Design review of the part built by this model. Coordinates are the model's own, in mm. A direction names the side the tool comes from. Coordinates: 2 decimals unless noted, no trailing zeros. Loops run counter-clockwise (first coordinate to the right, second up) from the corner with the lowest first, then second, coordinate; pieces in that order, holes last. Notation, with made-up numbers: (-4, 4.25) - (5, 4.25) arc R8 cw to (5, 11.25) - close; hole circle Ø8 at (44, 43.25). An arc over 180 degrees is marked (long way). One line per question, with ' | ' between items.
from build123d import *

# Parameters (mm, degrees)
F1_DEPTH = 76.2
F2_R     = 12.7
F3_DEPTH = 76.201
F5_DEPTH = 25.401
F6_R     = 38.1
F7_R     = 19.05
F8_DEPTH = 6.35


with BuildPart() as f1:
    # F0 (on Front) → F1 (new body, symmetric)
    with BuildSketch(Plane.XZ):
        Polygon((-76.2, 0), (0, 0), (0, 152.4), (-25.4, 152.4), (-25.4, 25.4), (-76.2, 25.4), align=None)
    extrude(amount=F1_DEPTH, both=True)

    # F2 (on face) → F3 (cut, through all)
    with BuildSketch(Plane.YZ):
        with Locations((0, 101.6)):
            Circle(F2_R)
    extrude(amount=-F3_DEPTH, mode=Mode.SUBTRACT)

    # F4 (on face) → F5 (cut, through all)
    with BuildSketch(Plane.XY.offset(25.4)):
        with BuildLine():
            ThreePointArc((-63.5, -6.35), (-59.009872, -4.490128), (-57.15, 0))
            ThreePointArc((-57.15, 0), (-59.009872, 4.490128), (-63.5, 6.35))
            ThreePointArc((-63.5, 6.35), (-69.85, 0), (-63.5, -6.35))
        make_face()
        with BuildLine():
            ThreePointArc((-63.5, -6.35), (-69.85, 0), (-63.5, 6.35))
            Line((-63.5, 6.35), (-76.2, 6.35))
            Line((-76.2, 6.35), (-76.2, -6.35))
            Line((-76.2, -6.35), (-63.5, -6.35))
        make_face()
    extrude(amount=-F5_DEPTH, mode=Mode.SUBTRACT)

    # F6
    f6_edges = [f1.edges().sort_by_distance(p)[0] for p in [
        (-12.7, -76.2, 152.4),
        (-12.7, 76.2, 152.4),
    ]]
    fillet(f6_edges, radius=F6_R)

    # F7 (on face) → F8 (cut)
    with BuildSketch(Plane(origin=(-25.4, 0, 0), x_dir=(0, -1, 0), z_dir=(-1, 0, 0))):
        with Locations((0, 101.6)):
            Circle(F7_R)
    extrude(amount=-F8_DEPTH, mode=Mode.SUBTRACT)


solid = f1.part
Q1. Take a section at B-B (y = 23). Give the boundary of the cut face in (x, z), plus the area to 3 significant figures.
Returned:
outline: (-76.2, 0) - (0, 0) - (0, 152.4) - (-25.4, 152.4) - (-25.4, 25.4) - (-76.2, 25.4) - close | area: 5,160 mm²
Q2. For pin 1 (1.5 mm diameter, centred on y = -17.5, z = 109.5, fed in from -X); pin 2 (23 mm diameter, centred on y = 0, z = 101.6, fed in from -X); pin 3 (12 mm diameter, centred on x = -13, y = -54.5, fed in from +Z); pin 4 (12 mm diameter, centred on x = -55.5, y = 10.5, fed in from +Z), all flat-tipped, find the tip position at first contact; note any pin that passes through.
Returned:
pin 1: stops at x = -25.4 | pin 2: passes through | pin 3: stops at z = 150.95 | pin 4: stops at z = 25.4
Q3. To check wall thickness, follow line 1 along Z through (x, y) = (-20.75, 0); line 2 along Y through (x, z) = (-21, 101); line 3 along X through (y, z) = (14, 58). State the ranges of each line that lie inside material, in increasing order.
Returned:
line 1: z = 0 to 82.55, 120.65 to 152.4 | line 2: y = -76.2 to -19.04, 19.04 to 76.2 | line 3: x = -25.4 to 0
Q4. Take a section at D-D (z = 40). Give the boundary of the cut face in (x, y).
Returned:
outline: (-25.4, -76.2) - (0, -76.2) - (0, 76.2) - (-25.4, 76.2) - close
Q5. Draft analysis for pull direction Z (two halves, no side actions). For faces 1 (the flat face through (-22, 76.2, 45)), 2 (the flat face through (-19.05, -12.4, 97.6)), 3 (the flat face through (-13, -1, 152.4)), state which applies: +Z half, -Z half, draft (parallel to the pull), parting line (faces both ways), or undercut.
Returned:
face 1: draft | face 2: undercut | face 3: +Z half
Q6. Take a section at A-A (z = 101.6). Give the boundary of the cut face in (x, y).
Returned:
outline: (-25.4, -76.2) - (0, -76.2) - (0, -12.7) - (-19.05, -12.7) - (-19.05, -19.05) - (-25.4, -19.05) - close; (-25.4, 19.05) - (-19.05, 19.05) - (-19.05, 12.7) - (0, 12.7) - (0, 76.2) - (-25.4, 76.2) - close
Q7. Take a section at C-C (x = -54). Give the boundary of the cut face in (y, z), plus the area to 3 significant figures.
Returned:
outline: (-76.2, 0) - (76.2, 0) - (76.2, 25.4) - (-76.2, 25.4) - close | area: 3,870 mm²
Q8. Tool access review of faces 4 (the flat face through (-25.4, -1, 76)), 5 (the cylindrical face through (-22.269, 2.48, 120.488)), 6 (the flat face through (-70, -6.35, 13)): name each direction out of +Z, -Z, +X, -X, +Y, -Y from which nothing blocks a thin tool from reaching the whole face with its end or side.
Returned:
face 4: +Z, -X, +Y, -Y | face 5: -X | face 6: +Z, -Z, -X
